Part model, mm, in its own coordinate system. Face numbers are marked on the shaded views. A direction names the side the tool comes from. Round coordinates to 2 decimals unless told otherwise and drop trailing zeros. Return JSON: item names as keys, results as strings. Group by question number.
(1) Drop flat-ended pins along their axis: pin 1 Ø7 at (x, z) = (0, 0) entering from -Y; pin 2 Ø4 at (y, z) = (3, -23.5) entering from +X; pin 3 Ø6 at (x, y) = (9.5, 13.5) entering from -Z; pin 4 Ø3 at (x, y) = (51.5, 9) entering from +Z. Give the stop position or say it passes through.
(2) Drill centre lines: L1, parallel to X at y = 3.8, z = 0; L2, parallel to Z at x = 0, y = 3.25; L3, parallel to X at y = 1.45, z = 0. Where is each one in solid material? Low to high. Write a range as from..to.
(3) Saw through at A-A (z = 0). State how many separate pieces and enclosed holes the cut face has, plus the area to 3 significant figures.
(4) Tool access for the marked faces 1, 2 and 3: list every direction of +Z, -Z, +X, -X, +Y, -Y with a clear straight run to the whole face (end or side of a thin tool).
from build123d import *

# Parameters (mm, degrees)
ESQUISSE1_R             = 4.5
ESQUISSE1_R_2           = 2.5
BOSS_EXTRU_1_DEPTH      = 15
ESQUISSE2_OUTSIDE_W     = 172.858
ESQUISSE2_OUTSIDE_H     = 199.18
ENL_V_MAT_EXTRU_1_DEPTH = 103.80323738
CONG_1_R                = 5
ENL_V_MAT_EXTRU_2_DEPTH = 9
ESQUISSE3_W             = 26.279593634
ESQUISSE3_H             = 20.5
ENL_V_MAT_EXTRU_3_DEPTH = 10
CONG_2_R                = 5
CONG_3_R                = 0.5
ESQUISSE5_R             = 7.505553499
BOSS_EXTRU_2_DEPTH      = 1.5
CHANFREIN1_SIZE         = 3.5


with BuildPart() as part:
    # Esquisse1 → Boss.-Extru.1 (new body)
    with BuildSketch(Plane(origin=(0, 0, 0), x_dir=(1, 0, 0), z_dir=(0, 1, 0))):
        Polygon((-65.032881815, 0), (0, -78.193541284), (65.032881815, 0), (0, 78.193541284), align=None)
        with Locations(Location((0, 0, 0), (0, 0, 270))):
            Circle(ESQUISSE1_R, mode=Mode.SUBTRACT)
        with Locations(Location((-47.5, 0, 0), (0, 0, 270))):
            Circle(ESQUISSE1_R_2, mode=Mode.SUBTRACT)
        with Locations(Location((47.5, 0, 0), (0, 0, 270))):
            Circle(ESQUISSE1_R_2, mode=Mode.SUBTRACT)
    extrude(amount=BOSS_EXTRU_1_DEPTH)

    # Esquisse2 outside → Enlèv. mat.-Extru.1 (cut, through all)
    with BuildSketch(Plane(origin=(0, 15, 0), x_dir=(1, 0, 0), z_dir=(0, 1, 0))):
        Rectangle(ESQUISSE2_OUTSIDE_W, ESQUISSE2_OUTSIDE_H)
        Polygon((0, 65.032881815), (-78.193541284, 0), (0, -65.032881815), (78.193541284, 0), align=None, mode=Mode.SUBTRACT)
    extrude(amount=-ENL_V_MAT_EXTRU_1_DEPTH, mode=Mode.SUBTRACT)

    # Congé1
    cong_1_edges = [part.edges().sort_by_distance(p)[0] for p in [
        (35.504282094, 7.5, -35.504282094),
        (35.504282094, 7.5, 35.504282094),
        (-35.504282094, 7.5, 35.504282094),
        (-35.504282094, 7.5, -35.504282094),
        (0, 7.5, -65.032881815),
        (0, 7.5, 65.032881815),
        (65.032881815, 7.5, 0),
        (-65.032881815, 7.5, 0),
    ]]
    fillet(cong_1_edges, radius=CONG_1_R)

    # Esquisse4 → Enlèv. mat.-Extru.2 (cut)
    with BuildSketch(Plane(origin=(0, 15, 0), x_dir=(1, 0, 0), z_dir=(0, 1, 0))):
        Polygon((6.5, 3.75277675), (0, 7.505553499), (-6.5, 3.75277675), (-6.5, -3.75277675), (0, -7.505553499), (6.5, -3.75277675), align=None)
    extrude(amount=-ENL_V_MAT_EXTRU_2_DEPTH, mode=Mode.SUBTRACT)

    # Esquisse3 → Enlèv. mat.-Extru.3 (cut)
    with BuildSketch(Plane(origin=(0, 15, 0), x_dir=(1, 0, 0), z_dir=(0, 1, 0))):
        with Locations((-50.389796817, 0)):
            Rectangle(ESQUISSE3_W, ESQUISSE3_H)
        with Locations((50.389796817, 0)):
            Rectangle(ESQUISSE3_W, ESQUISSE3_H)
    extrude(amount=-ENL_V_MAT_EXTRU_3_DEPTH, mode=Mode.SUBTRACT)

    # Congé2
    cong_2_edges = [part.edges().sort_by_distance(p)[0] for p in [
        (46.153054923, 15, -22.700524447),
        (-46.153054923, 15, 22.700524447),
        (-19.174121952, 15, -49.08593292),
        (19.174121952, 15, 49.08593292),
        (46.153054923, 15, 22.700524447),
        (19.174121952, 15, -49.08593292),
        (-46.153054923, 15, -22.700524447),
        (-19.174121952, 15, 49.08593292),
        (0, 15, -63.529593634),
        (0, 15, 63.529593634),
        (-35.489387791, 15, 35.489387791),
        (35.489387791, 15, 35.489387791),
        (35.489387791, 15, -35.489387791),
        (-35.489387791, 15, -35.489387791),
    ]]
    fillet(cong_2_edges, radius=CONG_2_R)

    # Congé3
    cong_3_edges = [part.edges().sort_by_distance(p)[0] for p in [
        (-19.174121952, 0, -49.08593292),
        (-49.08593292, 0, -19.174121952),
        (49.08593292, 0, 19.174121952),
        (19.174121952, 0, 49.08593292),
        (-19.174121952, 0, 49.08593292),
        (-49.08593292, 0, 19.174121952),
        (19.174121952, 0, -49.08593292),
        (49.08593292, 0, -19.174121952),
        (-63.529593634, 0, 0),
        (63.529593634, 0, 0),
        (0, 0, -63.529593634),
        (0, 0, 63.529593634),
        (-35.489387791, 0, 35.489387791),
        (35.489387791, 0, 35.489387791),
        (35.489387791, 0, -35.489387791),
        (-35.489387791, 0, -35.489387791),
    ]]
    fillet(cong_3_edges, radius=CONG_3_R)

    # Esquisse5 → Boss.-Extru.2 (add)
    with BuildSketch(Plane(origin=(0, 15, 0), x_dir=(1, 0, 0), z_dir=(0, 1, 0))):
        Circle(ESQUISSE5_R)
        Polygon((6.2, 3.579571669), (0, 7.159143338), (-6.2, 3.579571669), (-6.2, -3.579571669), (0, -7.159143338), (6.2, -3.579571669), align=None, mode=Mode.SUBTRACT)
    extrude(amount=-BOSS_EXTRU_2_DEPTH)

    # Chanfrein1
    chanfrein1_edges = [part.edges().sort_by_distance(p)[0] for p in [
        (-47.5, 0, -2.5),
        (47.5, 0, -2.5),
    ]]
    chamfer(chanfrein1_edges, length=CHANFREIN1_SIZE)


solid = part.part
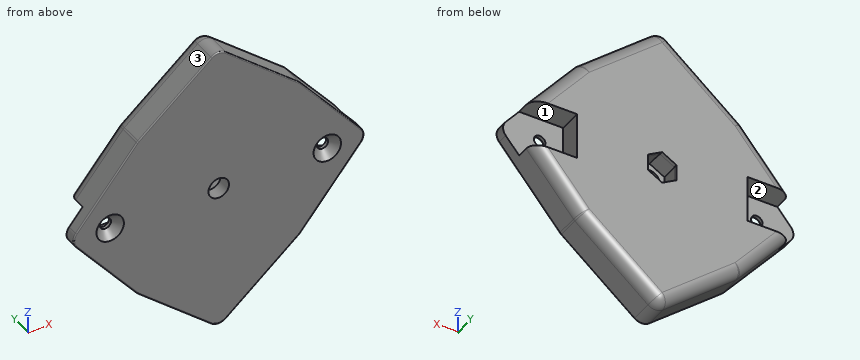
Computed values:
{
 "1": {"pin 1": "through", "pin 2": "x = 47.15", "pin 3": "z = -58.75", "pin 4": "z = 18.08"},
 "2": {"L1": "-63.53..-50, -45..-4.5, 4.5..45, 50..63.53", "L2": "-63.53..-4.5, 4.5..63.53", "L3": "-63.53..-52.05, -42.95..-4.5, 4.5..42.95, 52.05..63.53"},
 "3": {"separate pieces": "4", "enclosed holes": "0", "area": "1,140 mm2"},
 "4": {"face 1": "+X, +Y", "face 2": "-X, +Y", "face 3": "+Z, -X, +Y, -Y"}
}
